Build history of the part. All positions in model axes, mm. A direction names the side the tool comes from. Round coordinates to 2 decimals unless told otherwise and drop trailing zeros. Write each loop counter-clockwise with the first axis right and the second up, starting at its lowest first coordinate (ties: lowest second). Pieces come first, ordered by that corner, then holes. Notation, with made-up numbers: (62.25, -1.5) -> (84.25, -1.5) arc R22 ccw to (84.25, 20.5) -> close; hole circle Ø7 at (-5, 50). An arc over 180 degrees is marked (long way). Return JSON: item names as keys, results as strings.
from build123d import *

# Parameters (mm, degrees)
F0_R      = 5
F1_DEPTH  = 10.1
F2_R      = 4.8
F3_DEPTH  = 3
F5_DEPTH  = 5
F6_R      = 6
F7_DEPTH  = 3
F8_R      = 5
F9_DEPTH  = 5
F10_R     = 2.5
F11_DEPTH = 80


with BuildPart() as f1:
    # F0 (on Right) → F1 (new body)
    with BuildSketch(Plane.YZ):
        Circle(F0_R)
    extrude(amount=-F1_DEPTH)

    # F2 (on face) → F3 (join)
    with BuildSketch(Plane.YZ):
        Circle(F2_R)
    extrude(amount=F3_DEPTH)

    # F4 (on face) → F5 (join)
    with BuildSketch(Plane.YZ.offset(3)):
        Polygon((-4.565071, -1.483282), (0, -4.8), (4.565071, -1.483282), (2.821369, 3.883282), (-2.821369, 3.883282), align=None)
    extrude(amount=F5_DEPTH)

    # F6 (on face) → F7 (join)
    with BuildSketch(Plane(origin=(-10.1, 0, 0), x_dir=(0, -1, 0), z_dir=(-1, 0, 0))):
        Circle(F6_R)
    extrude(amount=F7_DEPTH)

    # F8 (on face) → F9 (join)
    with BuildSketch(Plane(origin=(-13.1, 0, 0), x_dir=(0, -1, 0), z_dir=(-1, 0, 0))):
        Circle(F8_R)
    extrude(amount=F9_DEPTH)

    # F10 (on face) → F11 (cut)
    with BuildSketch(Plane.YZ.offset(8)):
        Circle(F10_R)
    extrude(amount=-F11_DEPTH, mode=Mode.SUBTRACT)


solid = f1.part
Q1. Saw through at B-B on z = 1.75. List the corners of the cut face in (x, y).
Verdict:
{"outline": "(-18.1, -4.68) -> (-13.1, -4.68) -> (-13.1, -5.74) -> (-10.1, -5.74) -> (-10.1, -4.68) -> (0, -4.68) -> (0, -4.47) -> (3, -4.47) -> (3, -3.51) -> (8, -3.51) -> (8, -1.79) -> (-18.1, -1.79) -> close; (-18.1, 1.79) -> (8, 1.79) -> (8, 3.51) -> (3, 3.51) -> (3, 4.47) -> (0, 4.47) -> (0, 4.68) -> (-10.1, 4.68) -> (-10.1, 5.74) -> (-13.1, 5.74) -> (-13.1, 4.68) -> (-18.1, 4.68) -> close"}
Q2. Wall check: L1, parallel to Z at x = -7.75, y = 0; L2, parallel to Z at x = -11.75, y = 0; L3, parallel to X at y = 4.75, z = 1. Give the ranges that are in metal, low to high.
Verdict:
{"L1": "z = -5 to -2.5, 2.5 to 5", "L2": "z = -6 to -2.5, 2.5 to 6", "L3": "x = -18.1 to 0"}
Q3. Two-plate mould, pull along Z, no slides. Class faces 6 (the flat face through (-18.1, -2, -2)), 7 (the flat face through (5.465, 3.705, 1.162)), 8 (the cylindrical face through (-4.87, -0.54, -2.44)), 9 (the cylindrical face through (-4.98, -1.08, -4.88)): +Z half, -Z half, draft (parallel to the pull), parting line (faces both ways), or undercut.
Verdict:
{"face 6": "draft", "face 7": "+Z half", "face 8": "undercut", "face 9": "parting line"}
Q4. Saw through at A-A on y = -1.5. List the corners of the cut face in (x, z), then the cut area to 3 significant figures.
Verdict:
{"outline": "(-18.1, -4.77) -> (-13.1, -4.77) -> (-13.1, -5.81) -> (-10.1, -5.81) -> (-10.1, -4.77) -> (0, -4.77) -> (0, -4.56) -> (3, -4.56) -> (3, -3.71) -> (8, -3.71) -> (8, -2) -> (-18.1, -2) -> close; (-18.1, 2) -> (8, 2) -> (8, 3.88) -> (3, 3.88) -> (3, 4.56) -> (0, 4.56) -> (0, 4.77) -> (-10.1, 4.77) -> (-10.1, 5.81) -> (-13.1, 5.81) -> (-13.1, 4.77) -> (-18.1, 4.77) -> close", "area": "140 mm²"}
Q5. 3-axis set-ups, long thin cutter, end or side, ignore diameter. For faces 1 (the flat face through (5.46, -3.68, 1.24)), 2 (the flat face through (3, 4, 1)), 3 (the flat face through (-13.1, 4, 4)), 4 (the flat face through (3, 2.6, -3.5)), 5 (the flat face through (-10.1, 4, 4)): which of +Z, -Z, +X, -X, +Y, -Y reach the whole face in a straight line?
Verdict:
{"face 1": "+Z, +X, -Y", "face 2": "+Z, +X, +Y", "face 3": "-X", "face 4": "-Z, +X, +Y", "face 5": "+X"}
Q6. Saw through at C-C on x = 6.25. List the corners of the cut face in (y, z).
Verdict:
{"outline": "(-4.57, -1.48) -> (0, -4.8) -> (4.57, -1.48) -> (2.82, 3.88) -> (-2.82, 3.88) -> close; hole circle Ø5 at (0, 0)"}
Q7. Saw through at D-D on z = 4.25. List the corners of the cut face in (x, y), then the cut area to 3 significant figures.
Verdict:
{"outline": "(-18.1, -2.63) -> (-13.1, -2.63) -> (-13.1, -4.24) -> (-10.1, -4.24) -> (-10.1, -2.63) -> (0, -2.63) -> (0, -2.23) -> (3, -2.23) -> (3, 2.23) -> (0, 2.23) -> (0, 2.63) -> (-10.1, 2.63) -> (-10.1, 4.24) -> (-13.1, 4.24) -> (-13.1, 2.63) -> (-18.1, 2.63) -> close", "area": "118 mm²"}
Q8. Pin check, flat tips, straight feed: pin 1 Ø1 at (x, y) = (-14, 4) entering from -Z; pin 2 Ø2 at (x, y) = (-3.5, -4) entering from -Z; pin 3 Ø6 at (x, z) = (-3.5, -2) entering from +Y. Stop position of each tip, or through.
Verdict:
{"pin 1": "stops at z = -3.57", "pin 2": "stops at z = -4", "pin 3": "stops at y = 5"}
